Job drawing, mm, ordinate dimensions from the low corner. One solid piece. Give positions to 0.01 mm unless a question says otherwise; leave off trailing zeros. Write each loop counter-clockwise with the first axis right and the second up, starting at its lowest first coordinate (ties: lowest second). Pieces come first, ordered by that corner, then holes. Notation, with made-up numbers: (53, 40.5) -> (60, 40.5) arc R32 ccw to (60, 79.5) -> close; hole circle Ø10 at (78, -40). An arc over 180 degrees is marked (long way). Put each result on its own line as item: value. Start each with the question number.
Item 1: Slice it at C-C, the plane z = 1.2. List the corners of the cut face in (x, y), plus the area to 3 significant figures.
Item 2: Flat gauge pin, fed straight in: pin 1 Ø0.9 at (x, z) = (64, 1) entering from +Y. Where does the tip first touch, or does it go through?
Item 3: Drill centre lines: line 1 along X through (y, z) = (18.5, 1.6); line 2 along X through (y, z) = (19.25, 2.95); line 3 along Y through (x, z) = (40, 2.4). Where is each one in solid material? Low to high.
Item 4: Slice it at A-A, the plane y = 17. List the corners of the cut face in (x, z).
Item 5: Slice it at D-D, the plane x = 49.5. List the corners of the cut face in (y, z).
Item 6: Slice it at B-B, the plane x = 4. List the corners of the cut face in (y, z), plus the area to 3 significant figures.
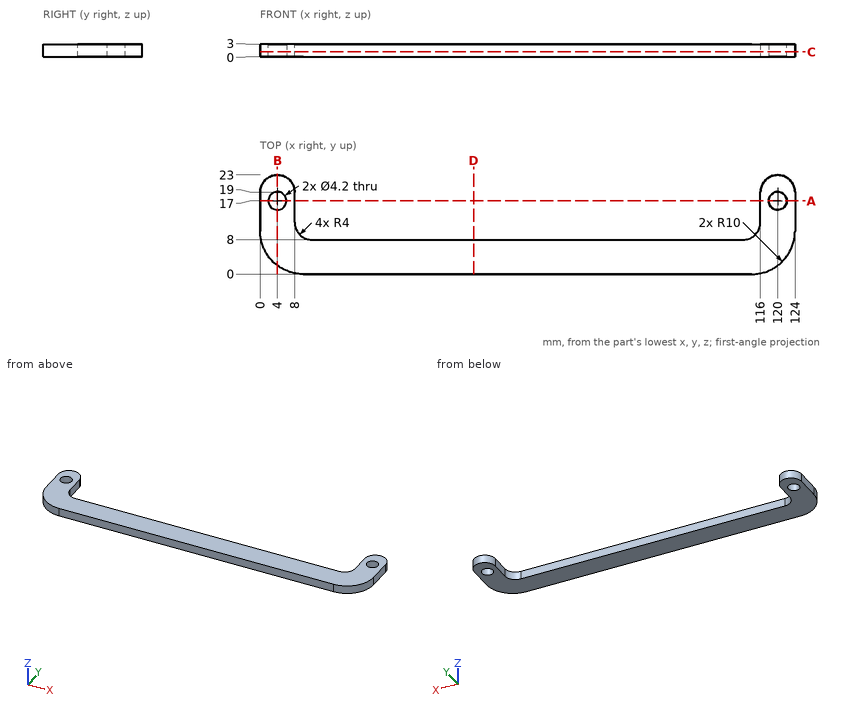
Values follow:
1. outline: (0, 10) arc R10 ccw to (10, 0) -> (114, 0) arc R10 ccw to (124, 10) -> (124, 19) arc R4 ccw to (116, 19) -> (116, 12) arc R4 cw to (112, 8) -> (12, 8) arc R4 cw to (8, 12) -> (8, 19) arc R4 ccw to (0, 19) -> close; hole circle Ø4.2 at (4, 17); hole circle Ø4.2 at (120, 17)
1. area: 1,150 mm2
2. pin 1: y = 8
3. line 1: 0 to 2.53, 5.47 to 8, 116 to 118.53, 121.47 to 124
3. line 2: 0.01 to 7.99, 116.01 to 123.99
3. line 3: 0 to 8
4. outline: (0, 0) -> (1.9, 0) -> (1.9, 3) -> (0, 3) -> close; (6.1, 0) -> (8, 0) -> (8, 3) -> (6.1, 3) -> close; (116, 0) -> (117.9, 0) -> (117.9, 3) -> (116, 3) -> close; (122.1, 0) -> (124, 0) -> (124, 3) -> (122.1, 3) -> close
5. outline: (0, 0) -> (8, 0) -> (8, 3) -> (0, 3) -> close
6. outline: (2, 0) -> (14.9, 0) -> (14.9, 3) -> (2, 3) -> close; (19.1, 0) -> (23, 0) -> (23, 3) -> (19.1, 3) -> close
6. area: 50.4 mm2
